from build123d import *

# Parameters (mm, degrees)
CHAMFER1_SIZE = 0.1125
FILLET1_R     = 0.1125


with BuildPart() as part:
    # Sketch3 → Revolve1 (revolve)
    with BuildSketch(Plane(origin=(0, 0, 0), x_dir=(0, 0, -1), z_dir=(1, 0, 0))):
        Polygon((3, 7), (1.5, 7), (1.5, 5.525), (-3, 5.525), (-3, 4), (3, 4), align=None)
    revolve(axis=Axis((0, 0, -3), (0, 0, 1)))

    # Chamfer1
    chamfer1_edges = [part.edges().sort_by_distance(p)[0] for p in [
        (0, -4, 3),
        (0, -5.525, 3),
        (0, -7, -1.5),
        (0, -7, -3),
    ]]
    chamfer(chamfer1_edges, length=CHAMFER1_SIZE)

    # Fillet1
    fillet1_edges = [part.edges().sort_by_distance(p)[0] for p in [
        (0, -5.525, -1.5),
    ]]
    fillet(fillet1_edges, radius=FILLET1_R)


solid = part.part
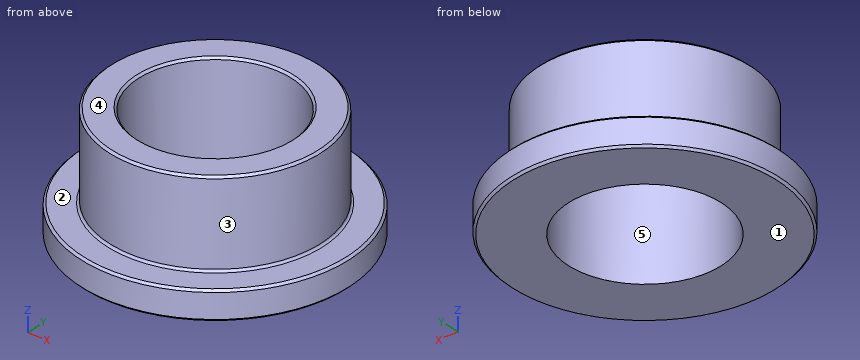
Input: part model. Units: mm. Frame: model coordinates. Face numbers are marked on the shaded views. A direction names the side the tool comes from. Coordinates: 2 decimals unless noted, no trailing zeros. Order: outer loops, then holes, each group sorted by start corner. A loop starts at its lowest first (then second) coordinate and runs counter-clockwise, first axis right, second up.
1. Cut plane C-C, the plane z = 0.15. Return loops of the section in (x, y) (3 decimals).
Checked values:
outline: circle Ø11.05 at (0, 0); hole circle Ø8 at (0, 0)
2. Contact query for a flat-ended pin moving along its axis: P1, Ø1, axis at x = 0, y = 2.5, coming from the +Z side. Output: stop coordinate, or through.
Checked values:
P1: passes through
3. Ray query, line 1 along X through (y, z) = (0, -1) (3 decimals); line 2 along Y through (x, z) = (-1.75, 1.6). Return the intervals inside material, ascending.
Checked values:
line 1: x = -5.525 to -4, 4 to 5.525
line 2: y = -5.24 to -3.6, 3.6 to 5.24
4. Access query for the marked faces 1 and 2. Directions: +Z, -Z, +X, -X, +Y, -Y. A direction counts if a zero-diameter tool reaches every point of the face in a straight line with its end or side. Return the directions, or none.
Checked values:
face 1: -Z, +X, -X, +Y, -Y
face 2: +Z
5. Draft query along Y for the marked faces 3, 4 and 5. Return one class per face: +Y half, -Y half, draft (parallel to the pull), parting line (faces both ways), or undercut.
Checked values:
face 3: parting line
face 4: draft
face 5: undercut
